Autodesk Inventor part; units mm, degrees
ref_plane "C3_XY" through (32.5, 0, 0) normal (-1, 0, 0) x (0, 0, -1)
ref_plane "C3_YZ" through (32.5, 0, 0) normal (0, 0, -1) x (0, -1, 0)
ref_plane "C3_ZX" through (32.5, 0, 0) normal (0, -1, 0) x (-1, 0, 0)
sketch "Sketch_1" plane through (0, 0, 0) normal (0, 0, 1) x (1, 0, 0)
  line L0 (32.5, 0) -> (0, 0)
  line L1 (0, 0) -> (0, 3)
  line L2 (0, 3) -> (0.5485, 3.95)
  line L3 (0.5485, 3.95) -> (31.9515, 3.95)
  line L4 (31.9515, 3.95) -> (32.5, 3)
  line L5 (32.5, 3) -> (32.5, 0)
  line L6 (32.5, 0) -> (0, 0)
revolve "Revolution1" add sketch "Sketch_1" angle 360 about axis through (32.5, 0, 0) along (1, 0, 0)
sketch "Sketch_2" plane through (0, 0, 0) normal (1, 0, 0) x (0, 1, 0)
  line L0 (6, 6) -> (-6, 6)
  line L1 (-6, 6) -> (-6, -6)
  line L2 (-6, -6) -> (6, -6)
  line L3 (6, -6) -> (6, 6)
  line L4 (-1.7321, 3) -> (-3.4641, 0)
  line L5 (-3.4641, 0) -> (-1.7321, -3)
  line L6 (-1.7321, -3) -> (1.7321, -3)
  line L7 (1.7321, -3) -> (3.4641, 0)
  line L8 (3.4641, 0) -> (1.7321, 3)
  line L9 (1.7321, 3) -> (-1.7321, 3)
extrude "Extrusion1" cut sketch "Sketch_2" along normal blind 32.5
sketch "Sketch3" plane through (0, 0, 0) normal (-1, 0, 0) x (0, 0, 1)
  point P0 (0, 0)
hole "Hole1" at (0, 0, 0) direction (1, 0, 0) diameter 2.459 depth 8.2901 tip angle 120 countersink diameter 3 countersink angle 90
sketch "Sketch4" plane through (32.5, 0, 0) normal (1, 0, 0) x (0, 0, -1)
  point P0 (0, 0)
hole "Hole2" at (32.5, 0, 0) direction (-1, 0, 0) diameter 2.459 depth 8.2901 tip angle 120 countersink diameter 3 countersink angle 90
ref_plane "C3_XY" through (32.5, 0, 0) normal (-1, 0, 0) x (0, 0, -1)
ref_plane "C3_YZ" through (32.5, 0, 0) normal (0, 0, -1) x (0, -1, 0)
ref_plane "C3_ZX" through (32.5, 0, 0) normal (0, -1, 0) x (-1, 0, 0)
properties part number "ABLSBF6-32.5-M3-N3" material "Aluminum 2014-T4"
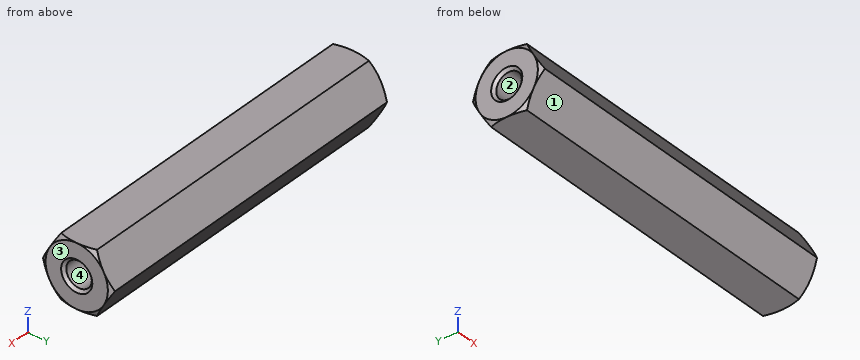
Work out the finished part from the listing and answer in its coordinate system (mm). Face numbers are marked on the shaded views. Give positions to 0.01 mm unless a question says otherwise; leave off trailing zeros. Order: outer loops, then holes, each group sorted by start corner. A loop starts at its lowest first (then second) coordinate and runs counter-clockwise, first axis right, second up. Notation, with made-up numbers: (-13.75, 81.25) -> (-5.75, 81.25) arc R7 cw to (-5.75, 89.25) -> close; hole circle Ø1 at (-40, 63). An arc over 180 degrees is marked (long way). Answer as a JSON object with one key per item and string values. Group by question number.
1. Section A-A on x = 29 is taken. Determine the outline of the cut face in (y, z).
2. The mould has two halves that part along Y. Classify the marked faces 1, 2, 3 and 4: released by +Y, released by -Y, zero draft, split by the parting line, or undercut.
3. Flat-ended cylindrical pins translate along their axes: pin 1 Ø4 at (x, y) = (25, 2) entering from +Z; pin 2 Ø1.5 at (x, z) = (5, 2.5) entering from +Y; pin 3 Ø2 at (y, z) = (0, 0) entering from -X; pin 4 Ø1.5 at (x, z) = (14.5, -2) entering from -Y. Find the tip coordinate at first contact, or state that the pin passes through.
4. Consider line 1 along Z through (x, y) = (28.75, 0); line 2 along Y through (x, z) = (29, 0.35); line 3 along X through (y, z) = (0.5, 0.2). Determine where each line is inside the solid, lowest interval first. Write a range as [from, to].
5. Section B-B on x = 10 is taken. Determine the outline of the cut face in (y, z).
Result sheet:
{
 "1": {"outline": "(-3.46, 0) -> (-1.73, -3) -> (1.73, -3) -> (3.46, 0) -> (1.73, 3) -> (-1.73, 3) -> close; hole circle Ø2.46 at (0, 0)"},
 "2": {"face 1": "released by -Y", "face 2": "undercut", "face 3": "zero draft", "face 4": "undercut"},
 "3": {"pin 1": "stops at z = 3", "pin 2": "stops at y = 2.45", "pin 3": "stops at x = 8.42", "pin 4": "stops at y = -2.74"},
 "4": {"line 1": "z = [-3, -1.23], [1.23, 3]", "line 2": "y = [-3.26, -1.18], [1.18, 3.26]", "line 3": "x = [8.69, 23.81]"},
 "5": {"outline": "(-3.46, 0) -> (-1.73, -3) -> (1.73, -3) -> (3.46, 0) -> (1.73, 3) -> (-1.73, 3) -> close"}
}
